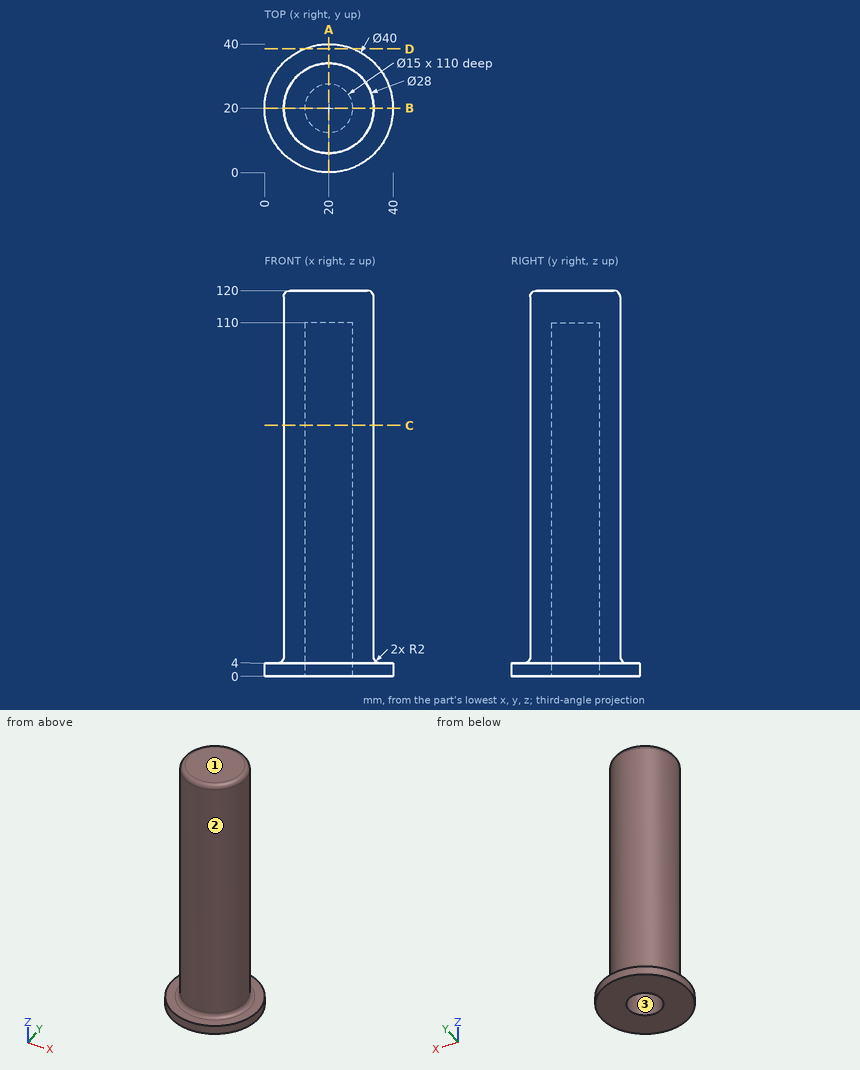
The figure shows three views and two pictorial views of one solid part (mm, origin at its lowest corner). Answer the questions. A direction names the side the tool comes from. Round coordinates to 2 decimals unless told otherwise and drop trailing zeros. Write each loop counter-clockwise with the first axis right and the second up, starting at its lowest first coordinate (ties: lowest second). Pieces come first, ordered by that corner, then holes. Notation, with made-up numbers: (31, -11.75) - (88, -11.75) arc R30 ccw to (88, 16.25) - close; hole circle Ø6 at (40, 26.5). An arc over 180 degrees is marked (long way). Answer in a Markdown table with one row per item. Add a question column.
1. A cutting plane is placed at D-D, the plane y = 38.5. Determine the outline of the cut face in (x, z).
2. Given pin 1 (8 mm diameter, centred on x = 21.5, z = 71.5, fed in from -Y); pin 2 (6 mm diameter, centred on x = 13.5, z = 32.5, fed in from -Y); pin 3 (12 mm diameter, centred on x = 20, y = 20, fed in from -Z), each flat-ended and moving along its own axis, determine where each tip first touches the part or whether it passes through.
3. For the marked faces 1, 2 and 3, determine the directions among +Z, -Z, +X, -X, +Y, -Y from which every point of the face is accessible in a straight line to the end or side of a thin tool.
4. Find the intervals of material crossed by line 1 along Y through (x, z) = (20, 33); line 2 along Z through (x, y) = (7.5, 33), in increasing order. Write a range as from..to.
5. A cutting plane is placed at C-C, the plane z = 78. Determine the outline of the cut face in (x, y).
6. A cutting plane is placed at A-A, the plane x = 20. Determine the outline of the cut face in (y, z), and give its area (3 significant figures).
Worked out:
| question | item | result |
|---|---|---|
| 1 | outline | (12.4, 0) - (27.6, 0) - (27.6, 4) - (12.4, 4) - close |
| 2 | pin 1 | y = 6 |
| 2 | pin 2 | y = 6.44 |
| 2 | pin 3 | z = 110 |
| 3 | face 1 | +Z, +X, -X, +Y, -Y |
| 3 | face 2 | +Z |
| 3 | face 3 | -Z |
| 4 | line 1 | 6..12.5, 27.5..34 |
| 4 | line 2 | 0..4 |
| 5 | outline | circle Ø28 at (20, 20); hole circle Ø15 at (20, 20) |
| 6 | outline | (0, 0) - (12.5, 0) - (12.5, 110) - (27.5, 110) - (27.5, 0) - (40, 0) - (40, 4) - (36, 4) arc R2 cw to (34, 6) - (34, 118) arc R2 ccw to (32, 120) - (8, 120) arc R2 ccw to (6, 118) - (6, 6) arc R2 cw to (4, 4) - (0, 4) - close |
| 6 | area | 1,760 mm^2 |
